from build123d import *

# Parameters (mm, degrees)
SKETCH_1_R          = 20
EXTRUDE_1_DEPTH     = 2
SKETCH_2_R          = 18.5
EXTRUDE_2_DEPTH     = 7
SKETCH_3_R          = 10
CUT_EXTRUDE_1_DEPTH = 30.681644159
SKETCH_4_R          = 16.638615911
SKETCH_4_R_2        = 14.166384124
CUT_EXTRUDE_2_DEPTH = 0.5


with BuildPart() as part:
    # 草图1 → 凸台-拉伸1 (new body)
    with BuildSketch(Plane.XY):
        Circle(SKETCH_1_R)
    extrude(amount=EXTRUDE_1_DEPTH)

    # 草图2 → 凸台-拉伸2 (add)
    with BuildSketch(Plane.XY.offset(2)):
        Circle(SKETCH_2_R)
    extrude(amount=EXTRUDE_2_DEPTH)

    # 草图3 → 切除-拉伸1 (cut, through all)
    with BuildSketch(Plane.XY.offset(9)):
        Circle(SKETCH_3_R)
    extrude(amount=-CUT_EXTRUDE_1_DEPTH, mode=Mode.SUBTRACT)

    # 草图4 → 切除-拉伸2 (cut)
    with BuildSketch(Plane(origin=(0, 0, 0), x_dir=(-1, 0, 0), z_dir=(0, 0, -1))):
        Circle(SKETCH_4_R)
        Circle(SKETCH_4_R_2, mode=Mode.SUBTRACT)
    extrude(amount=-CUT_EXTRUDE_2_DEPTH, mode=Mode.SUBTRACT)


solid = part.part
Geometry check sheet. Reference: the model listing, model coordinates, mm. A direction names the side the tool comes from. Coordinates: 2 decimals unless noted, no trailing zeros. Write each loop counter-clockwise with the first axis right and the second up, starting at its lowest first coordinate (ties: lowest second). Pieces come first, ordered by that corner, then holes. Notation, with made-up numbers: (78, -25.5) -> (122, -25.5) arc R29 ccw to (122, -5.5) -> close; hole circle Ø7 at (85.5, 75.25). An arc over 180 degrees is marked (long way). One line per question, with ' | ' between items.
1. Draft check along Y on faces 3 (the cylindrical face through (-2.17, -9.76, 4.56)), 4 (the flat face through (6, -18, 2)), 5 (the cylindrical face through (3.07, -13.83, 0.25)), 6 (the cylindrical face through (-4.01, -18.06, 5.45)). Enter one of: +Y half, -Y half, draft (parallel to the pull), parting line (faces both ways), or undercut.
Answers:
face 3: undercut | face 4: draft | face 5: undercut | face 6: parting line
2. Cross-section at D-D on y = -16. Record the cut outline in (x, z).
Answers:
outline: (-12, 0) -> (-4.57, 0) -> (-4.57, 0.5) -> (4.57, 0.5) -> (4.57, 0) -> (12, 0) -> (12, 2) -> (9.29, 2) -> (9.29, 9) -> (-9.29, 9) -> (-9.29, 2) -> (-12, 2) -> close
3. Depth check by flat-ended pin: pin 1 Ø3 at (y, z) = (13.5, 7.5) entering from -X; pin 2 Ø4 at (x, z) = (-14, 2) entering from +Y; pin 3 Ø1.5 at (x, z) = (8.5, 5) entering from -Y. Enter the tip coordinate at first touch or a pass-through.
Answers:
pin 1: stops at x = -14.08 | pin 2: stops at y = 16 | pin 3: stops at y = -16.8
4. Set-up check for faces 1 (the flat face through (8, -8, 9)), 2 (the flat face through (-12.2, 7.5, 0.5)): record each of +Z, -Z, +X, -X, +Y, -Y from which the full face is reachable in a straight line by a thin tool's end or side.
Answers:
face 1: +Z, +X, -X, +Y, -Y | face 2: -Z
5. Cross-section at A-A on x = 0. Record the cut outline in (y, z).
Answers:
outline: (-20, 0) -> (-16.64, 0) -> (-16.64, 0.5) -> (-14.17, 0.5) -> (-14.17, 0) -> (-10, 0) -> (-10, 9) -> (-18.5, 9) -> (-18.5, 2) -> (-20, 2) -> close; (10, 0) -> (14.17, 0) -> (14.17, 0.5) -> (16.64, 0.5) -> (16.64, 0) -> (20, 0) -> (20, 2) -> (18.5, 2) -> (18.5, 9) -> (10, 9) -> close
6. Thickness scan on probe 1 along Y at (x, z) = (0, 0.1); probe 2 along Y at (x, z) = (0, 4.25); probe 3 along Z at (x, y) = (18, 4.5). Record the ranges inside material, lowest first. Write a range as from..to.
Answers:
probe 1: y = -20..-16.64, -14.17..-10, 10..14.17, 16.64..20 | probe 2: y = -18.5..-10, 10..18.5 | probe 3: z = 0..2
7. Cross-section at C-C on z = 1.25. Record the cut outline in (x, y).
Answers:
outline: circle Ø40 at (0, 0); hole circle Ø20 at (0, 0)
